Autodesk Inventor part; units mm, degrees
ref_plane "Work Plane1" through (10, 0, 0) normal (0, -0.5, -0.866) x (1, 0, 0)
ref_plane "YZ Plane" through (0, 0, 0) normal (1, 0, 0) x (0, 1, 0)
ref_plane "XZ Plane" through (0, 0, 0) normal (0, 1, 0) x (-1, 0, 0)
sketch "Skizze1" plane through (0, 0, 0) normal (0, 0, 1) x (1, 0, 0)
  line L0 (0.866, 0) -> (15.5, 0)
  line L1 (20, 1.7321) -> (20, 3)
  line L2 (20, 3) -> (0, 3)
  line L3 (20, 1.7321) -> (16.5, 1.7321)
  line L4 (16.5, 1.7321) -> (15.5, 0)
  line L5 (0, 1.5) -> (0.866, 0)
  line L6 (0, -0.6) -> (0, 3.6)
  line L7 (0, 1.5) -> (0, 3)
  point P0 (0, 0)
  dimension "d0" = 3.5
  dimension "d1" = 60
  dimension "d2" = 6
  dimension "d3" = 3.4641
  dimension "d4" = 20
  dimension "d5" = 60
  dimension "d7" = 3
revolve "Körper" add sketch "Skizze1" angle 360 about axis through (0.866, 0, 0) along (1, 0, 0)
sketch "Skizze2" plane through (20, 0, 0) normal (1, 0, 0) x (0, 0, -1)
  circle A0 centre (0, 0) radius 1.7321
  circle A1 centre (0, 0) radius 3
  line L0 (1.7321, 0) -> (0.866, -1.5)
  line L1 (0.866, -1.5) -> (-0.866, -1.5)
  line L2 (-0.866, -1.5) -> (-1.7321, 0)
  line L3 (-1.7321, 0) -> (-0.866, 1.5)
  line L4 (-0.866, 1.5) -> (0.866, 1.5)
  line L5 (0.866, 1.5) -> (1.7321, 0)
extrude "Loch" add sketch "Skizze2" against normal blind 3.5 contours L5 A0 | A0 L0 | L4 A0 | A0 L1 | L3 A0 | A0 L2
chamfer "Fase1" distance 1.5 angle 45 1 edges at (0, -3, 0) measured on face at (0, 2.4709, -0.2393)
thread "Gewinde"
chamfer "Fase2" distance 0.6135 angle 45 1 edges at (20, -3, 0) measured on face at (13.8332, 2.9612, -0.4812)
ref_plane "Work Plane1" through (10, 0, 0) normal (0, -0.5, -0.866) x (1, 0, 0)
equation "\"d0\" = INTI"
equation "\"d2\" = NND"
equation "\"d3\" = 1.1547 * SW"
equation "\"d4\" = NLG"
equation "\"d5\" = 0.5 * ANG"
equation "\"d7\" = SPD"
equation "\"d8\" = INTI"
equation "\"d10\" = -0.5 * SPD + 0.5 * NND"
equation "\"d11\" = FAWI"
equation "\"d33\" = -0.5 * SPD + 0.5 * NND"
equation "\"d14\" = NLG"
equation "\"d12\" = -0.5 * GD1 + 0.5 * NND"
equation "\"d13\" = FAWI"
equation "\"d34\" = -0.5 * GD1 + 0.5 * NND"
equation "\"NND\" = 6"
equation "\"NLG\" = 20"
equation "\"INTI\" = 3.5"
equation "\"FAWI\" = 45deg"
equation "\"SW\" = 3"
equation "\"GD1\" = THREADDIA - 1.2269 * PTC"
equation "\"ANG\" = 120deg"
equation "\"FAWI1\" = 45deg"
equation "\"SPD\" = 3"
equation "\"GUL\" = 0.61345 * PTC"
equation "\"TOA\" = 30deg"
equation "\"THREADDIA\" = 6"
equation "\"PTC\" = 1"
equation "\"GAL\" = 0.61345 * PTC"
equation "\"E0\" = 1.155 * SW"
properties part number "ISO 4029 - M6 x 20" material "Edelstahl, 440C"
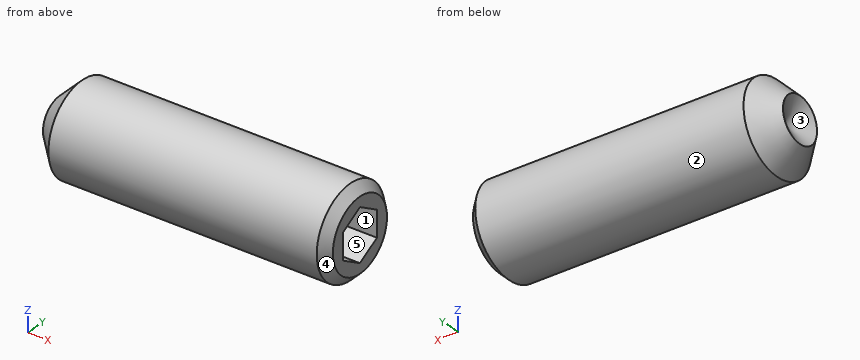
Work out the finished part from the listing and answer in its coordinate system (mm). Face numbers are marked on the shaded views. A direction names the side the tool comes from. Coordinates: 2 decimals unless noted, no trailing zeros. Write each loop counter-clockwise with the first axis right and the second up, starting at its lowest first coordinate (ties: lowest second). Pieces come first, ordered by that corner, then holes. Notation, with made-up numbers: M -21,61 L 20,61 A17 cw 20,92 Z; hole C 89,-36.5 d8. An arc over 180 degrees is marked long. Answer as CSV lines item,"result". Start each with the question number.
Item 1: Section A-A on x = 3 is taken. Write down the section's boundary in (y, z).
Item 2: Determine the mould class of the marked faces 3, 4 and 5 for opening direction Y: released by +Y, released by -Y, zero draft, split by the parting line, or undercut.
Item 3: Flat-ended cylindrical pins translate along their axes: P1, Ø1, axis at x = 17.5, y = 1.5, coming from the -Z side; P2, Ø2, axis at x = 3.5, z = -1.5, coming from the -Y side. Find the tip coordinate at first contact, or state that the pin passes through.
Item 4: A tool of negligible diameter and unlimited length cuts with its end or side. For the marked faces 1 and 2, from which of +Z, -Z, +X, -X, +Y, -Y can it reach the whole face along a straight path? Write none if from no direction.
Item 5: Consider L1, parallel to Z at x = 2, y = 0.15; L2, parallel to Y at x = 19.25, z = -0.55; L3, parallel to Z at x = 17.5, y = -1.4. Determine where each line is inside the solid, lowest interval first.
Checks:
1,outline,"C 0,0 d6"
2,face 3,"undercut"
2,face 4,"split by the parting line"
2,face 5,"undercut"
3,P1,"stops at z = -2.83"
3,P2,"stops at y = -2.96"
4,face 1,"+X"
4,face 2,"+X, -X"
5,L1,"z = -3 to 3"
5,L2,"y = -2.95 to -1.5, 1.5 to 2.95"
5,L3,"z = -2.65 to -0.92, 0.92 to 2.65"
